Part model, mm, in its own coordinate system. A direction names the side the tool comes from. Coordinates: 2 decimals unless noted, no trailing zeros. Order: outer loops, then holes, each group sorted by start corner. A loop starts at its lowest first (then second) coordinate and runs counter-clockwise, first axis right, second up.
1) Wall check: L1, parallel to Y at x = 11.5, z = 12.25; L2, parallel to Y at x = 24.5, z = 4; L3, parallel to Y at x = 45, z = 12. Give the ranges that are in metal, low to high.
2) Cut at D-D (y = 41.5). List the corners of the cut face in (x, z).
3) Cut at A-A (y = 5). List the corners of the cut face in (x, z).
4) Cut at C-C (x = 24.6). List the corners of the cut face in (y, z).
5) Tool access for faces 4 (the flat face through (42, 0, 9)), 5 (the flat face through (7, 0, 9)), 6 (the flat face through (7, 22, 9)): list every direction of +Z, -Z, +X, -X, +Y, -Y with a clear straight run to the whole face (end or side of a thin tool).
6) Pin check, flat tips, straight feed: pin 1 Ø5 at (x, z) = (39.5, 7.5) entering from +Y; pin 2 Ø2 at (x, z) = (14.5, 5) entering from +Y; pin 3 Ø1.8 at (x, y) = (24.6, 5) entering from -Z; pin 4 Ø7.5 at (x, z) = (38, 6) entering from -Y. Stop position of each tip, or through.
7) Mould opens along Y. For faces 1 (the flat face through (16.1, 35.5, 11.3)), 2 (the cylindrical face through (23.1, 5.07, 8.82)), 3 (the cylindrical face through (15.38, 46.59, 11.65)) say: +Y half, -Y half, draft (parallel to the pull), parting line (faces both ways), or undercut.
8) Cut at B-B (x = 37.7). List the corners of the cut face in (y, z), and give its area (3 significant figures).
Autodesk Inventor part; units mm, degrees
ref_plane "YZ Plane" through (0, 0, 0) normal (1, 0, 0) x (0, 1, 0)
ref_plane "XZ Plane" through (0, 0, 0) normal (0, 1, 0) x (-1, 0, 0)
ref_plane "XY Plane" through (0, 0, 0) normal (0, 0, 1) x (1, 0, 0)
sketch "スケッチ1" plane through (0, 0, 0) normal (0, 0, 1) x (1, 0, 0)
  line L0 (0, 0) -> (49.2, 0)
  line L1 (49.2, 0) -> (49.2, 20)
  line L2 (49.2, 20) -> (0, 20)
  line L3 (0, 20) -> (0, 0)
  line L4 (15, 0) -> (19.5921, -3.4)
  line L5 (19.5921, -3.4) -> (29.6079, -3.4)
  line L6 (29.6079, -3.4) -> (34.2, 0)
  dimension "d0" = 49.2
  dimension "d1" = 20
  dimension "d2" = 15
  dimension "d3" = 15
  dimension "d4" = 3.4
extrude "押し出し1" add sketch "スケッチ1" along normal blind 17.4
sketch "スケッチ2" plane through (0, 20, 0) normal (0, 1, 0) x (1, 0, 0)
  circle A0 centre (13.5, -8.7) radius 8.1
  line L0 (0, 0) -> (0, -17.4)
  circle A1 centre (13.5, -8.7) radius 6
  circle A2 centre (13.5, -8.7) radius 3.5
  dimension "d7" = 16.2
  dimension "d8" = 13.5
  dimension "d9" = 12
  dimension "d10" = 7
extrude "押し出し2" add sketch "スケッチ2" along normal blind 2 contours A0
extrude "押し出し3" add sketch "スケッチ2" along normal blind 15.5 contours A1
extrude "押し出し4" add sketch "スケッチ2" along normal blind 38 contours A2
sketch "スケッチ3" plane through (13.5, 58, 8.7) normal (0, 1, 0) x (1, 0, 0)
  circle A0 centre (0, 0) radius 0.5
  point P0 (-13.5, 8.7)
  dimension "d17" = 1
extrude "押し出し5" add sketch "スケッチ3" along normal blind 77.5
sketch "スケッチ4" plane through (0, 0, 17.4) normal (0, 0, 1) x (1, 0, 0)
  line L0 (0, 0) -> (15, 0)
  line L1 (34.2, 0) -> (49.2, 0)
  line L2 (49.2, 0) -> (49.2, 20)
  line L3 (0, 20) -> (0, 0)
  point P0 (11.5, 5)
  point P1 (37.7, 5)
  dimension "d20" = 5
  dimension "d21" = 5
  dimension "d22" = 11.5
  dimension "d23" = 11.5
hole "穴1" at (11.5, 5, 17.4) at (37.7, 5, 17.4) direction (0, 0, -1) diameter 4 end through all
sketch "スケッチ5" plane through (0, 0, 17.4) normal (0, 0, 1) x (1, 0, 0)
  circle A0 centre (11.5, 5) radius 2
  circle A1 centre (37.7, 5) radius 2
  line L0 (29.6079, -3.4) -> (34.2, 0)
  line L1 (34.2, 0) -> (49.2, 0)
  line L2 (49.2, 0) -> (49.2, 20)
  line L3 (49.2, 20) -> (0, 20)
  line L4 (0, 20) -> (0, 0)
  line L5 (0, 0) -> (15, 0)
  line L6 (15, 0) -> (19.5921, -3.4)
  line L7 (19.5921, -3.4) -> (29.6079, -3.4)
  circle A2 centre (24.6, 5) radius 1.5
  dimension "d31" = 3
extrude "押し出し6" cut sketch "スケッチ5" against normal blind 40 contours A2
properties part number "Z-15HNJS55-B" material "ABS プラスチック"
Geometry check:
1. L1: y = 0 to 3, 7 to 35.5
1. L2: y = -3.4 to 3.5, 6.5 to 20
1. L3: y = 0 to 20
2. outline: circle Ø7 at (13.5, 8.7)
3. outline: (0, 0) - (9.5, 0) - (9.5, 17.4) - (0, 17.4) - close; (13.5, 0) - (23.1, 0) - (23.1, 17.4) - (13.5, 17.4) - close; (26.1, 0) - (35.7, 0) - (35.7, 17.4) - (26.1, 17.4) - close; (39.7, 0) - (49.2, 0) - (49.2, 17.4) - (39.7, 17.4) - close
4. outline: (-3.4, 0) - (3.5, 0) - (3.5, 17.4) - (-3.4, 17.4) - close; (6.5, 0) - (20, 0) - (20, 17.4) - (6.5, 17.4) - close
5. face 4: +Z, -Z, +X, -Y
5. face 5: +Z, -Z, -X, -Y
5. face 6: +Y
6. pin 1: stops at y = 20
6. pin 2: stops at y = 58
6. pin 3: passes through
6. pin 4: stops at y = 0
7. face 1: +Y half
7. face 2: undercut
7. face 3: draft
8. outline: (0, 0) - (3, 0) - (3, 17.4) - (0, 17.4) - close; (7, 0) - (20, 0) - (20, 17.4) - (7, 17.4) - close
8. area: 278 mm2
